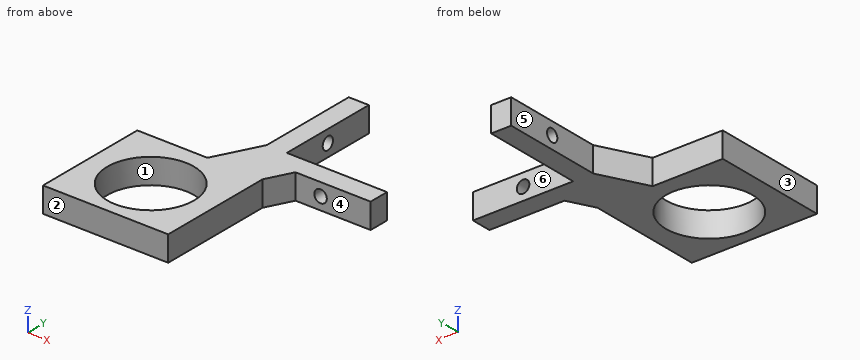
from build123d import *

# Parameters (mm, degrees)
SKETCH1_W           = 27.94
SKETCH1_H           = 27.94
SKETCH1_W_2         = 5.08
SKETCH1_H_2         = 66.04
BOSS_EXTRUDE1_DEPTH = 6.35
SKETCH2_R           = 1.5875
CUT_EXTRUDE1_DEPTH  = 12.7
SKETCH3_W           = 6.35
SKETCH3_H           = 5.08
BOSS_EXTRUDE2_DEPTH = 25.4
SKETCH4_R           = 1.5875
CUT_EXTRUDE2_DEPTH  = 25.4
SKETCH5_R           = 10.99185
CUT_EXTRUDE3_DEPTH  = 25.4
BOSS_EXTRUDE3_DEPTH = 6.35
SKETCH8_W           = 31.75
SKETCH8_H           = 29.21
SKETCH8_R           = 10.99185
BOSS_EXTRUDE4_DEPTH = 6.35
SKETCH9_W           = 4.445
SKETCH9_H           = 27.94
CUT_EXTRUDE4_DEPTH  = 6.35


with BuildPart() as part:
    # Sketch1 → Boss-Extrude1 (new body)
    with BuildSketch(Plane.XY):
        with Locations((-16.51, -19.05)):
            Rectangle(SKETCH1_W, SKETCH1_H)
        Rectangle(SKETCH1_W_2, SKETCH1_H_2)
    extrude(amount=BOSS_EXTRUDE1_DEPTH)

    # Sketch2 → Cut-Extrude1 (cut)
    with BuildSketch(Plane.ZY.offset(2.54)):
        with Locations((3.175, 20.32)):
            Circle(SKETCH2_R)
    extrude(amount=-CUT_EXTRUDE1_DEPTH, mode=Mode.SUBTRACT)

    # Sketch3 → Boss-Extrude2 (add)
    with BuildSketch(Plane(origin=(2.54, 0, 0), x_dir=(0, 0, -1), z_dir=(1, 0, 0))):
        with Locations((-3.175, 5.08)):
            Rectangle(SKETCH3_W, SKETCH3_H)
    extrude(amount=BOSS_EXTRUDE2_DEPTH)

    # Sketch4 → Cut-Extrude2 (cut)
    with BuildSketch(Plane.XZ.offset(-2.54)):
        with Locations((15.24, 3.175)):
            Circle(SKETCH4_R)
    extrude(amount=-CUT_EXTRUDE2_DEPTH, mode=Mode.SUBTRACT)

    # Sketch5 → Cut-Extrude3 (cut)
    with BuildSketch(Plane.XY.offset(6.35)):
        with Locations((-10.16, -19.05)):
            Circle(SKETCH5_R)
    extrude(amount=-CUT_EXTRUDE3_DEPTH, mode=Mode.SUBTRACT)

    # Sketch6 → Boss-Extrude3 (add)
    with BuildSketch(Plane.XY.offset(6.35)):
        Polygon((-2.54, 7.62), (-8.89, -5.08), (-2.54, -5.08), align=None)
        Polygon((2.54, 2.54), (2.54, -10.16), (8.89, 2.54), align=None)
    extrude(amount=-BOSS_EXTRUDE3_DEPTH)

    # Sketch8 → Boss-Extrude4 (add)
    with BuildSketch(Plane.XY.offset(6.35)):
        with Locations((-10.16, -18.415)):
            Rectangle(SKETCH8_W, SKETCH8_H)
        with Locations((-10.16, -19.05)):
            Circle(SKETCH8_R, mode=Mode.SUBTRACT)
    extrude(amount=-BOSS_EXTRUDE4_DEPTH)

    # Sketch9 → Cut-Extrude4 (cut)
    with BuildSketch(Plane.XY.offset(6.35)):
        with Locations((-28.2575, -19.05)):
            Rectangle(SKETCH9_W, SKETCH9_H)
    extrude(amount=-CUT_EXTRUDE4_DEPTH, mode=Mode.SUBTRACT)


solid = part.part
Can you work these out from the model? Positions are in its coordinate system, mm. Face numbers are marked on the shaded views. A direction names the side the tool comes from. Give positions to 0.01 mm unless a question says otherwise; leave off trailing zeros. Order: outer loops, then holes, each group sorted by start corner. A loop starts at its lowest first (then second) coordinate and runs counter-clockwise, first axis right, second up. Notation, with made-up numbers: M 10,47.5 L 62,47.5 A5 ccw 62,56.5 Z; hole C 73.5,34.5 d2. An arc over 180 degrees is marked long. One line per item, written item: value.
Item 1: If we section it at C-C on y = 20.32: Write out the boundary of the cut face in (x, z), and give its area (3 significant figures).
Verdict:
outline: M -2.54,0 L 2.54,0 L 2.54,1.59 L -2.54,1.59 Z; M -2.54,4.76 L 2.54,4.76 L 2.54,6.35 L -2.54,6.35 Z
area: 16.1 mm2
Item 2: If we section it at B-B on z = 5.5: Write out the boundary of the cut face in (x, y) (3 decimals), and give its area (3 significant figures).
Verdict:
outline: M -26.035,-33.02 L 5.715,-33.02 L 5.715,-3.81 L 8.89,2.54 L 27.94,2.54 L 27.94,7.62 L 2.54,7.62 L 2.54,33.02 L -2.54,33.02 L -2.54,7.62 L -8.255,-3.81 L -26.035,-3.81 Z; hole C -10.16,-19.05 d21.984
area: 927 mm2
Item 3: If we mould it in two halves opening along Y, with no side actions, what happens to the marked faces 1, 2 and 3? For each: pulls with the +Y half, pulls with the -Y half, needs draft (parallel to the pull), parting line crosses it, or undercut.
Verdict:
face 1: undercut
face 2: pulls with the -Y half
face 3: needs draft
Item 4: For the marked faces 4, 5 and 6, which set-ups out of +Z, -Z, +X, -X, +Y, -Y let a thin tool reach every point of the face, with its end or its side?
Verdict:
face 4: +Z, -Z, +X, -Y
face 5: +Z, -Z, -X, +Y
face 6: +Z, -Z, +X, +Y
Item 5: For pin 1 (2.5 mm diameter, centred on y = 20.32, z = 3.175, fed in from -X); pin 2 (3 mm diameter, centred on y = 19.5, z = 4, fed in from -X); pin 3 (3 mm diameter, centred on y = 20.5, z = 4.5, fed in from +X), each with a flat end and sliding along its axis, tell me the tip position at first contact or that it passes through.
Verdict:
pin 1: through
pin 2: x = -2.54
pin 3: x = 2.54
Item 6: If we section it at A-A on x = 15.24: Write out the boundary of the cut face in (y, z).
Verdict:
outline: M 2.54,0 L 7.62,0 L 7.62,1.59 L 2.54,1.59 Z; M 2.54,4.76 L 7.62,4.76 L 7.62,6.35 L 2.54,6.35 Z
Item 7: Please list where these lines run through material, in increasing order: line 1 (Y direction, x = -1, z = 3.5); line 2 (X direction, y = 21.5, z = 1.75); line 3 (Y direction, x = -1, z = 6).
Verdict:
line 1: -33.02 to -25.13, -12.97 to 18.77, 21.87 to 33.02
line 2: -2.54 to 2.54
line 3: -33.02 to -25.13, -12.97 to 33.02
Item 8: If we section it at D-D on x = 0: State how many separate pieces and enclosed holes the cut face has, and give its area (3 significant figures).
Verdict:
separate pieces: 2
enclosed holes: 1
area: 358 mm2
